```python
from build123d import *

# Parameters (mm, degrees)
F0_W      = 70
F0_H      = 140
F1_DEPTH  = 10
F3_R      = 8
F4_DEPTH  = 9
F6_DEPTH  = 1.001
F6_TAPER  = -3
F8_W      = 30
F8_H      = 3
F9_DEPTH  = 7.5
F10_R     = 2
F11_DEPTH = 25
F7_W      = 12
F7_H      = 5
F12_DEPTH = 10


with BuildPart() as f1:
    # F0 (on Top) → F1 (new body)
    with BuildSketch(Plane.XY):
        Rectangle(F0_W, F0_H)
    extrude(amount=F1_DEPTH)

    # F3
    f3_edges = [f1.edges().sort_by_distance(p)[0] for p in [
        (35, 70, 5),
        (-35, 70, 5),
        (35, -70, 5),
        (-35, -70, 5),
    ]]
    fillet(f3_edges, radius=F3_R)

    # F2 (on face) → F4 (cut)
    with BuildSketch(Plane.XY.offset(10)):
        with BuildLine():
            Line((19.5, 60), (-19.5, 60))
            ThreePointArc((-19.5, 60), (-25.1568542495, 57.6568542495), (-27.5, 52))
            Line((-27.5, 52), (-27.5, -52))
            ThreePointArc((-27.5, -52), (-25.1568542495, -57.6568542495), (-19.5, -60))
            Line((-19.5, -60), (19.5, -60))
            ThreePointArc((19.5, -60), (25.1568542495, -57.6568542495), (27.5, -52))
            Line((27.5, -52), (27.5, 52))
            ThreePointArc((27.5, 52), (25.1568542495, 57.6568542495), (19.5, 60))
        make_face()
    extrude(amount=-F4_DEPTH, mode=Mode.SUBTRACT)

    # F5 (on face) → F6 (cut, through all)
    with BuildSketch(Plane.XY.offset(1)):
        with BuildLine():
            Line((-7.5, 45), (-16.5, 45))
            ThreePointArc((-16.5, 45), (-18.6213203436, 44.1213203436), (-19.5, 42))
            Line((-19.5, 42), (-19.5, 33))
            ThreePointArc((-19.5, 33), (-18.6213203436, 30.8786796564), (-16.5, 30))
            Line((-16.5, 30), (-7.5, 30))
            ThreePointArc((-7.5, 30), (-5.3786796564, 30.8786796564), (-4.5, 33))
            Line((-4.5, 33), (-4.5, 42))
            ThreePointArc((-4.5, 42), (-5.3786796564, 44.1213203436), (-7.5, 45))
        make_face()
    extrude(amount=-F6_DEPTH, taper=F6_TAPER, mode=Mode.SUBTRACT)

    # F8 (on face) → F9 (cut, through all)
    with BuildSketch(Plane(origin=(-35, 0, 0), x_dir=(0, -1, 0), z_dir=(-1, 0, 0))):
        with Locations((-37, 5.1784133364)):
            Rectangle(F8_W, F8_H)
    extrude(amount=-F9_DEPTH, mode=Mode.SUBTRACT)

    # F10 (on face) → F11 (cut)
    with BuildSketch(Plane(origin=(0, 70, 0), x_dir=(-1, 0, 0), z_dir=(0, 1, 0))):
        with Locations((-17, 5)):
            Circle(F10_R)
    extrude(amount=-F11_DEPTH, mode=Mode.SUBTRACT)

    # F7 (on face) → F12 (cut, through all)
    with BuildSketch(Plane.XZ.offset(70)):
        with Locations((0, 4.5)):
            Rectangle(F7_W, F7_H)
    extrude(amount=-F12_DEPTH, mode=Mode.SUBTRACT)


solid = f1.part
```
Design review of the part built by this model. Coordinates are the model's own, in mm. A direction names the side the tool comes from. Coordinates: 2 decimals unless noted, no trailing zeros. Order: outer loops, then holes, each group sorted by start corner. A loop starts at its lowest first (then second) coordinate and runs counter-clockwise, first axis right, second up.
1) Take a section at A-A, the plane x = 17. Give the boundary of the cut face in (y, z).
2) Take a section at D-D, the plane y = -4.5. Give the boundary of the cut face in (x, z).
3) Clearance check with flat-ended pins moving along their axes: pin 1 (12 mm diameter, centred on x = 22.5, y = 30.5, fed in from +Z); pin 2 (3.5 mm diameter, centred on x = -30.5, z = 4.5, fed in from +Y); pin 3 (2.5 mm diameter, centred on x = -3, z = 5.5, fed in from -Y); pin 4 (3.5 mm diameter, centred on x = -32.5, z = 6, fed in from -Y). State where each tip first meets the part, or that it passes through.
4) For faces 4 (the conical face through (-5.34, 44.12, 0.49)), 5 (the flat face through (0, -60, 8)), 6 (the flat face through (-31, 37, 3.678)), 7 (the flat face through (0, -65, 2)), list the 3-axis set-ups (+Z, -Z, +X, -X, +Y, -Y) from which the entire face can be reached by the end or side of a thin tool; tool diameter is ignored.
5) Take a section at C-C, the plane z = 5. Give the boundary of the cut face in (x, y).
6) Mouldability with a two-part tool opening along Z and no side actions: class faces 1 (the flat face through (27.5, -1, 6)), 2 (the conical face through (-18.66, 30.88, 0.49)), 3 (the flat face through (-31, 22, 5)) as +Z half, -Z half, draft (parallel to the pull), parting line (faces both ways), or undercut.
7) Take a section at B-B, the plane y = 50. Give the boundary of the cut face in (x, z).
8) Wall thickness on line 1 along Y through (x, z) = (9, 2.25); line 2 along X through (y, z) = (-60.5, 4.75); line 3 along X through (y, z) = (-20, 2): over which ranges is each line inside the solid? List them lowest first.
Returned:
1. outline: (-70, 0) - (70, 0) - (70, 3) - (60, 3) - (60, 1) - (-60, 1) - (-60, 10) - (-70, 10) - close; (60, 7) - (70, 7) - (70, 10) - (60, 10) - close
2. outline: (-35, 0) - (35, 0) - (35, 10) - (27.5, 10) - (27.5, 1) - (-27.5, 1) - (-27.5, 10) - (-35, 10) - close
3. pin 1: stops at z = 10
3. pin 2: stops at y = 69.81
3. pin 3: stops at y = 60
3. pin 4: stops at y = -69.07
4. face 4: -Z
4. face 5: +Z
4. face 6: -X
4. face 7: -Y
5. outline: (-35, -62) arc R8 ccw to (-27, -70) - (-6, -70) - (-6, -60) - (-19.5, -60) arc R8 cw to (-27.5, -52) - (-27.5, 22) - (-35, 22) - close; (-35, 52) - (-27.5, 52) arc R8 cw to (-19.5, 60) - (15, 60) - (15, 70) - (-27, 70) arc R8 ccw to (-35, 62) - close; (6, -70) - (27, -70) arc R8 ccw to (35, -62) - (35, 62) arc R8 ccw to (27, 70) - (19, 70) - (19, 60) - (19.5, 60) arc R8 cw to (27.5, 52) - (27.5, -52) arc R8 cw to (19.5, -60) - (6, -60) - close
6. face 1: draft
6. face 2: -Z half
6. face 3: undercut
7. outline: (-35, 0) - (35, 0) - (35, 10) - (27.5, 10) - (27.5, 1) - (-27.5, 1) - (-27.5, 3.68) - (-35, 3.68) - close; (-35, 6.68) - (-27.5, 6.68) - (-27.5, 10) - (-35, 10) - close
8. line 1: y = -70 to -60, 60 to 70
8. line 2: x = -35 to -6, 6 to 35
8. line 3: x = -35 to -27.5, 27.5 to 35
